Autodesk Fusion 360 part; units mm, degrees
sketch "Sketch1" plane through (0, 0, 0) normal (0, 1, 0) x (1, 0, 0)
  line L0 (0, 0) -> (179, 0) construction
  line L1 (179, 0) -> (179, -135) construction
  line L2 (179, -135) -> (0, -135) construction
  line L3 (0, -135) -> (0, 0) construction
  line L4 (0, -135) -> (0, -101.42)
  dimension "d1" = 179
  dimension "d2" = 135
  dimension "d3" = 101.42
sketch "Sketch2" plane through (0, 0, 0) normal (0, 1, 0) x (1, 0, 0)
  line L0 (0, 0) -> (160, 0) construction
  line L1 (179, -135) -> (0, -135) construction
  line L2 (0, -135) -> (0, 0) construction
  line L3 (0, -135) -> (0, -101.42)
  line L4 (80, -98.0476) -> (80, -100.5515)
  line L5 (40, -100.284) -> (40, -102.7879)
  line L6 (120, -95.8113) -> (120, -98.3152)
  line L7 (80, -100.5515) -> (70, -101.1106)
  line L8 (60, -99.1658) -> (70, -101.1106)
  line L9 (60, -99.1658) -> (40, -100.284)
  line L10 (40, -102.7879) -> (30, -103.347)
  line L11 (20, -101.4021) -> (30, -103.347)
  line L12 (160.0645, -96.0752) -> (149.3716, -96.6731)
  line L13 (140, -94.6931) -> (149.3716, -96.6731)
  line L14 (140, -94.6931) -> (120, -95.8113)
  line L15 (120, -98.3152) -> (110, -98.8743)
  line L16 (100, -96.9295) -> (110, -98.8743)
  line L17 (100, -96.9295) -> (80, -98.0476)
  line L18 (0, -101.42) -> (20, -101.4021)
  line L19 (160.0645, -96.0752) -> (179, -96.0752)
  line L20 (179, 0) -> (179, -135)
  line L21 (179, -96.0752) -> (179, -129.65)
  line L22 (179, -129.65) -> (174, -129.65)
  line L23 (0, -135) -> (5, -135)
  line L24 (5, -135) -> (5, -106.42)
  line L25 (174, -129.65) -> (174, -106.42)
  line L26 (5, -106.42) -> (20, -106.42)
  line L27 (20, -106.42) -> (20, -109.42)
  line L28 (20, -109.42) -> (40, -109.42)
  line L29 (40, -109.42) -> (40, -106.42)
  line L30 (40, -106.42) -> (60, -106.42)
  line L31 (60, -106.42) -> (60, -109.42)
  line L32 (60, -109.42) -> (80, -109.42)
  line L33 (80, -109.42) -> (80, -106.42)
  line L34 (80, -106.42) -> (100, -106.42)
  line L35 (100, -106.42) -> (100, -109.42)
  line L36 (100, -109.42) -> (120, -109.42)
  line L37 (120, -109.42) -> (120, -106.42)
  line L38 (120, -106.42) -> (140, -106.42)
  line L39 (140, -106.42) -> (140, -109.42)
  line L40 (140, -109.42) -> (160, -109.42)
  line L41 (160, -109.42) -> (160, -106.42)
  line L42 (160, -106.42) -> (174, -106.42)
  point P0 (179, 0)
  dimension "d4" = 179
  dimension "d5" = 135
  dimension "d6" = 101.42
  dimension "d7" = 129.65
  dimension "d8" = 5
  dimension "d9" = 5
  dimension "d10" = 5
  dimension "d12" = 15
  dimension "d13" = 109.42
  dimension "d14" = 20
  dimension "d15" = 20
  dimension "d16" = 3
  dimension "d17" = 20
  dimension "d18" = 3
  dimension "d19" = 20
  dimension "d20" = 3
  dimension "d21" = 20
  dimension "d22" = 20
  dimension "d23" = 3
  dimension "d24" = 20
  dimension "d25" = 3
revolve "Revolve1" add sketch "Sketch2" angle 360 about axis through (0, 0, 0) along (1, 0, 0)
sketch "Sketch3" plane through (0, 0, 0) normal (-1, 0, 0) x (0, -1, 0)
  circle A0 centre (0, 0) radius 135
  circle A1 centre (0, 0) radius 101.42
  line L0 (0, 0) -> (0, 166.4632) construction
  circle A2 centre (0, 122.55) radius 2
  dimension "d27" = 4
  dimension "d28" = 122.55
extrude "Extrude1" cut sketch "Sketch3" against normal blind 12 contours A2
pattern_circular "C-Pattern1" count 20 over 360 about axis through (1.75, 0, 0) along (1, 0, 0) of "Extrude1"
sketch "Sketch4" plane through (179, 0, 0) normal (1, 0, 0) x (0, 1, 0)
  circle A0 centre (0, 0) radius 96.0752
  circle A1 centre (0, 0) radius 129.65
  line L0 (0, 0) -> (0, 177.3715) construction
  circle A2 centre (0, 122.5) radius 2
  dimension "d33" = 4
  dimension "d34" = 122.5
extrude "Extrude2" cut sketch "Sketch4" against normal blind 13 contours A2
pattern_circular "C-Pattern2" count 20 over 360 about axis through (1.75, 0, 0) along (1, 0, 0) of "Extrude2"
Verification items for the finished model (mm, model axes). A direction names the side the tool comes from. Coordinates: 2 decimals unless noted, no trailing zeros. Loops run counter-clockwise (first coordinate to the right, second up) from the corner with the lowest first, then second, coordinate; pieces in that order, holes last. Notation, with made-up numbers: (-10.75, 37.5) - (41.25, 37.5) arc R21 ccw to (41.25, 71.5) - close; hole circle Ø8 at (-27, -28). An arc over 180 degrees is marked (long way). Put each result on its own line as item: value.
Item 1: Gauge pin test, flat ends, axial feed: pin 1 Ø2.5 at (y, z) = (-72.03, -99.15) entering from -X; pin 2 Ø1.5 at (x, z) = (20.5, -81.5) entering from +Y; pin 3 Ø2 at (y, z) = (91.5, 64) entering from -X; pin 4 Ø6 at (x, z) = (46, -66) entering from +Y. Record the tip position at first contact, or that the pin passes through.
Conclusion:
pin 1: passes through
pin 2: stops at y = 73.84
pin 3: stops at x = 0
pin 4: stops at y = 85.77
Item 2: Draft check along X on faces 1 (the face through (50.14, -31.966, 101.506)), 2 (the face through (56.53, 29.85, 94.77)), 3 (the face through (150.14, 106.82, -23.72)), 4 (the face through (2.54, 82.15, -107.13)). Enter one of: pulls with the +X half, pulls with the -X half, needs draft (parallel to the pull), parting line crosses it, or undercut.
Conclusion:
face 1: undercut
face 2: pulls with the -X half
face 3: undercut
face 4: needs draft
Item 3: Section check A-A (x = 86.5). Enter the section's corners in (y, z).
Conclusion:
outline: circle Ø212.84 at (0, 0); hole circle Ø195.37 at (0, 0)
Item 4: Scan lines: line 1 along Y through (x, z) = (3.15, 0); line 2 along X through (y, z) = (114.5, 59); line 3 along Y through (x, z) = (14, -43). Record each from-to range of solid material in increasing order.
Conclusion:
line 1: y = -135 to -124.55, -120.55 to -101.42, 101.42 to 120.55, 124.55 to 135
line 2: x = 0 to 5, 174 to 179
line 3: y = -97.35 to -91.84, 91.84 to 97.35
Item 5: Section check B-B (x = 26). Enter the section's corners in (y, z), then the cut area to 3 significant figures.
Conclusion:
outline: circle Ø218.84 at (0, 0); hole circle Ø205.14 at (0, 0)
area: 4,560 mm2
Item 6: Set-up check for faces 5 (the face through (179, 95, -20)), 6 (the face through (90.14, -31.966, 101.506)): record each of +Z, -Z, +X, -X, +Y, -Y from which the full face is reachable in a straight line by a thin tool's end or side.
Conclusion:
face 5: +Z, -Z, +X, +Y, -Y
face 6: none
